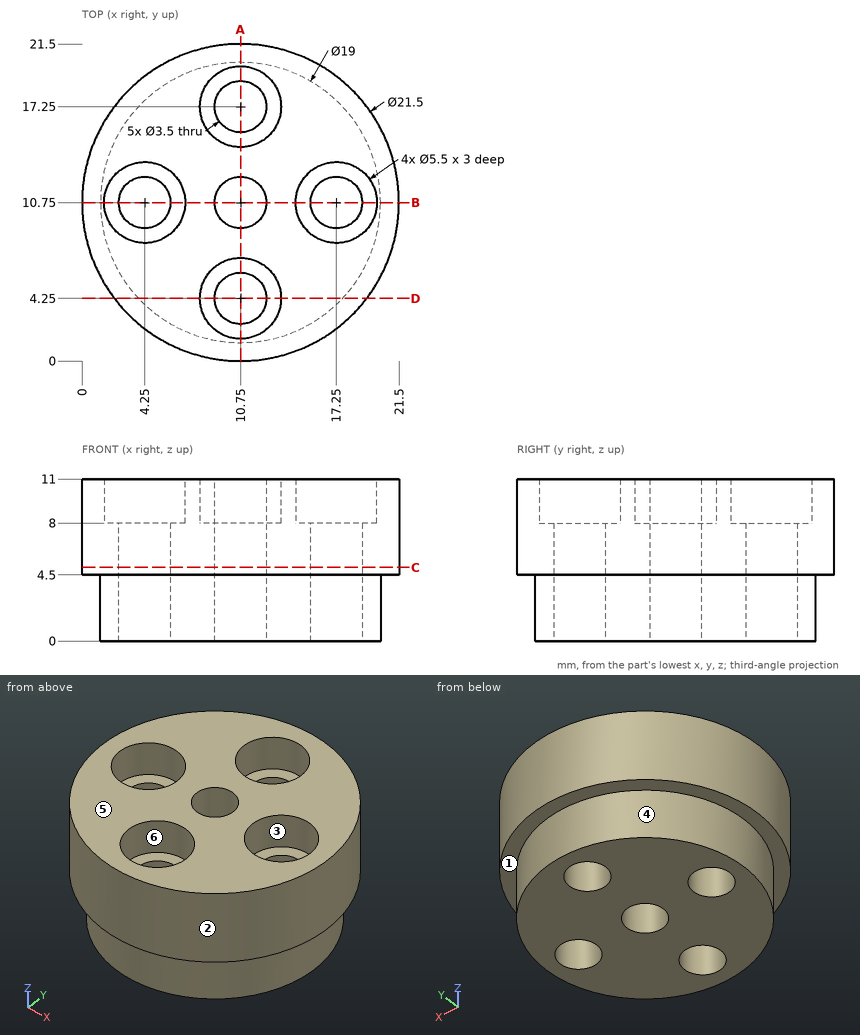
Design review of the part shown in the three views and the two pictorial views. Dimensions are in mm from the part's minimum x, y and z. A direction names the side the tool comes from. Round coordinates to 2 decimals unless told otherwise and drop trailing zeros. Loops run counter-clockwise (first coordinate to the right, second up) from the corner with the lowest first, then second, coordinate; pieces in that order, holes last. Notation, with made-up numbers: (-14.5, 6) - (30.5, 6) arc R22 ccw to (30.5, 13) - close; hole circle Ø11 at (41.5, 59.25). An arc over 180 degrees is marked (long way). Write each question's results on one line, items separated by ' | '. Start each with the question number.
Q1. Tool access review of the marked faces 1, 2 and 3: name each direction out of +Z, -Z, +X, -X, +Y, -Y from which nothing blocks a thin tool from reaching the whole face with its end or side.
Q2. Insertion check: P1, Ø3, axis at x = 16, z = 7.5, coming from the +Y side; P2, Ø5, axis at x = 10.75, y = 4.25, coming from the +Z side; P3, Ø6, axis at x = 10, y = 5.5, coming from the +Z side; P4, Ø3, axis at x = 17.25, y = 10.75, coming from the +Z side (3 decimals). Each pin has a flat end and moves straight along its axis. Give the tip position at first contact, or say it passes through.
Q3. Draft analysis for pull direction X (two halves, no side actions). For the marked faces 4, 5 and 6, state which applies: pulls with the +X half, pulls with the -X half, needs draft (parallel to the pull), parting line crosses it, or undercut.
Q4. Wall thickness on line 1 along Y through (x, z) = (10.75, 9.25); line 2 along Y through (x, z) = (10.75, 5.5); line 3 along X through (y, z) = (10, 7.25): over which ranges is each line inside the solid? List them lowest first. Write a range as [from, to].
Q5. Take a section at D-D on y = 4.25. Give the boundary of the cut face in (x, z).
Q6. Take a section at C-C on z = 5. Give the boundary of the cut face in (x, y), plus the area to 3 significant figures.
Q7. Take a section at A-A on x = 10.75. Give the boundary of the cut face in (y, z).
Data:
1) face 1: -Z | face 2: +Z, -Z | face 3: +Z
2) P1: stops at y = 20.82 | P2: stops at z = 8 | P3: stops at z = 11 | P4: passes through
3) face 4: parting line crosses it | face 5: needs draft | face 6: undercut
4) line 1: y = [0, 1.5], [7, 9], [12.5, 14.5], [20, 21.5] | line 2: y = [0, 2.5], [6, 9], [12.5, 15.5], [19, 21.5] | line 3: x = [0.03, 2.67], [5.83, 9.17], [12.33, 15.67], [18.83, 21.47]
5) outline: (2.19, 4.5) - (3.82, 4.5) - (3.82, 0) - (9, 0) - (9, 8) - (8, 8) - (8, 11) - (2.19, 11) - close; (12.5, 0) - (17.68, 0) - (17.68, 4.5) - (19.31, 4.5) - (19.31, 11) - (13.5, 11) - (13.5, 8) - (12.5, 8) - close
6) outline: circle Ø21.5 at (10.75, 10.75); hole circle Ø3.5 at (4.25, 10.75); hole circle Ø3.5 at (10.75, 4.25); hole circle Ø3.5 at (10.75, 10.75); hole circle Ø3.5 at (10.75, 17.25); hole circle Ø3.5 at (17.25, 10.75) | area: 315 mm²
7) outline: (0, 4.5) - (1.25, 4.5) - (1.25, 0) - (2.5, 0) - (2.5, 8) - (1.5, 8) - (1.5, 11) - (0, 11) - close; (6, 0) - (9, 0) - (9, 11) - (7, 11) - (7, 8) - (6, 8) - close; (12.5, 0) - (15.5, 0) - (15.5, 8) - (14.5, 8) - (14.5, 11) - (12.5, 11) - close; (19, 0) - (20.25, 0) - (20.25, 4.5) - (21.5, 4.5) - (21.5, 11) - (20, 11) - (20, 8) - (19, 8) - close
